Design review of the part built by this model. Coordinates are the model's own, in mm. Face numbers are marked on the shaded views. A direction names the side the tool comes from. Coordinates: 2 decimals unless noted, no trailing zeros. Write each loop counter-clockwise with the first axis right and the second up, starting at its lowest first coordinate (ties: lowest second). Pieces come first, ordered by that corner, then holes.
Q1. Take a section at A-A, the plane z = 7.75. Write out the cut boundary in (x, y).
Q2. For L1, parallel to Y at x = -13, z = 0.7; L2, parallel to X at y = -31, z = 13; L3, parallel to Y at x = 19.5, z = 3.75, list the stretches that pass through material, from the lowest coordinate up.
Q3. The part is to be moulded in two halves that separate along Y. For the marked faces 3, 4 and 5, say which applies: released by +Y, released by -Y, zero draft, split by the parting line, or undercut.
Q4. Take a section at B-B, the plane y = 16.5. Write out the cut boundary in (x, z), plus the area to 3 significant figures.
Q5. For the marked faces 1 and 2, list the 3-axis set-ups (+Z, -Z, +X, -X, +Y, -Y) from which the entire face can be reached by the end or side of a thin tool; tool diameter is ignored.
Q6. For pin 1 Ø3.5 at (x, z) = (-6, 7) entering from +Y; pin 2 Ø2 at (x, z) = (14.5, 9.5) entering from -Y; pin 3 Ø3 at (x, y) = (-12, 26.5) entering from +Z, all flat-tipped, find the tip position at first contact; note any pin that passes through.
Q7. Take a section at C-C, the plane x = -12.5. State how many separate pieces and enclosed holes the cut face has, plus the area to 3 significant figures.
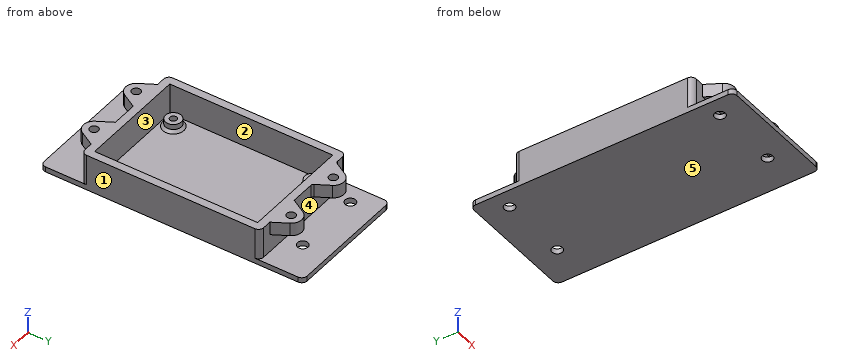
from build123d import *

# Parameters (mm, degrees)
SKETCH_1_W               = 40
SKETCH_1_H               = 100
SKETCH_1_R               = 2
EXTRUDE_1_DEPTH          = 2
SKETCH_2_W               = 47
SKETCH_2_H               = 68
SKETCH_2_W_2             = 41
SKETCH_2_H_2             = 62
EXTRUDE_2_DEPTH          = 11.8
SKETCH_3_W               = 7
SKETCH_3_H               = 100
EXTRUDE_3_DEPTH          = 2
SKETCH_4_R               = 3
SKETCH_4_R_2             = 1.3
EXTRUDE_4_DEPTH          = 3
SKETCH_5_R               = 1.3
CUT_EXTRUDE_1_DEPTH      = 3.5
SKETCH_6_R               = 1.65
EXTRUDE_5_DEPTH          = 5
CUT_EXTRUDE_2_DEPTH      = 2
FILLET_1_R               = 1
MIRROR_5_COPY_1_SKETCH_R = 1.65
MIRROR_5_COPY_1_DEPTH    = 5
MIRROR_5_COPY_2_DEPTH    = 2
FILLET_2_R               = 2
CHAMFER_1_SIZE           = 1


with BuildPart() as part:
    # 草图1 → 凸台-拉伸1 (new body)
    with BuildSketch(Plane.XY):
        Rectangle(SKETCH_1_W, SKETCH_1_H)
        with Locations((-13, 40)):
            Circle(SKETCH_1_R, mode=Mode.SUBTRACT)
        with Locations((13, 40)):
            Circle(SKETCH_1_R, mode=Mode.SUBTRACT)
        with Locations((-13, -40)):
            Circle(SKETCH_1_R, mode=Mode.SUBTRACT)
        with Locations((13, -40)):
            Circle(SKETCH_1_R, mode=Mode.SUBTRACT)
    extrude(amount=EXTRUDE_1_DEPTH)

    # 草图2 → 凸台-拉伸2 (add)
    with BuildSketch(Plane.XY.offset(2)):
        with Locations((3.5, -0.496887342)):
            Rectangle(SKETCH_2_W, SKETCH_2_H)
        with Locations((3.5, -0.496887342)):
            Rectangle(SKETCH_2_W_2, SKETCH_2_H_2, mode=Mode.SUBTRACT)
    extrude(amount=EXTRUDE_2_DEPTH)

    # 草图3 → 凸台-拉伸3 (add)
    with BuildSketch(Plane(origin=(0, 0, 0), x_dir=(-1, 0, 0), z_dir=(0, 0, -1))):
        with Locations((-23.5, 0)):
            Rectangle(SKETCH_3_W, SKETCH_3_H)
    extrude(amount=-EXTRUDE_3_DEPTH)

    # 草图4 → 凸台-拉伸4 (add)
    with BuildSketch(Plane.XY.offset(2)):
        with Locations(Location((-12.5, 26.003112658, 0), (0, 0, 180))):
            Circle(SKETCH_4_R)
        with Locations((-12.5, 26.003112658)):
            Circle(SKETCH_4_R_2, mode=Mode.SUBTRACT)
        with Locations(Location((19.5, 26.003112658, 0), (0, 0, 180))):
            Circle(SKETCH_4_R)
        with Locations((19.5, 26.003112658)):
            Circle(SKETCH_4_R_2, mode=Mode.SUBTRACT)
        with Locations(Location((19.5, -26.996887342, 0), (0, 0, 180))):
            Circle(SKETCH_4_R)
        with Locations((19.5, -26.996887342)):
            Circle(SKETCH_4_R_2, mode=Mode.SUBTRACT)
        with Locations(Location((-12.5, -26.996887342, 0), (0, 0, 180))):
            Circle(SKETCH_4_R)
        with Locations((-12.5, -26.996887342)):
            Circle(SKETCH_4_R_2, mode=Mode.SUBTRACT)
    extrude(amount=EXTRUDE_4_DEPTH)

    # 草图5 → 切除-拉伸1 (cut)
    with BuildSketch(Plane.XY.offset(5)):
        with Locations((-12.5, -26.996887342)):
            Circle(SKETCH_5_R)
        with Locations((19.5, -26.996887342)):
            Circle(SKETCH_5_R)
        with Locations((19.5, 26.003112658)):
            Circle(SKETCH_5_R)
        with Locations((-12.5, 26.003112658)):
            Circle(SKETCH_5_R)
    extrude(amount=-CUT_EXTRUDE_1_DEPTH, mode=Mode.SUBTRACT)

    # 草图6 → 凸台-拉伸5 (add)
    with BuildSketch(Plane.XY.offset(13.8)):
        with BuildLine():
            Line((-14.639528096, 33.503112658), (-1.360471904, 33.503112658))
            Line((-1.360471904, 33.503112658), (-4.535898385, 39.003112658))
            ThreePointArc((-4.535898385, 39.003112658), (-8, 41.003112658), (-11.464101615, 39.003112658))
            Line((-11.464101615, 39.003112658), (-14.639528096, 33.503112658))
        make_face()
        with Locations((-8, 37.003112658)):
            Circle(SKETCH_6_R, mode=Mode.SUBTRACT)
    extrude_5 = extrude(amount=-EXTRUDE_5_DEPTH)

    # 草图7 → 切除-拉伸2 (cut)
    with BuildSketch(Plane(origin=(0, 0, 8.8), x_dir=(-1, 0, 0), z_dir=(0, 0, -1))):
        Polygon((6.325684219, 39.903112658), (4.651368439, 37.003112658), (6.325684219, 34.103112658), (9.674315781, 34.103112658), (11.348631561, 37.003112658), (9.674315781, 39.903112658), align=None)
    cut_extrude_2 = extrude(amount=-CUT_EXTRUDE_2_DEPTH, mode=Mode.SUBTRACT)

    # 圆角1
    fillet_1_edges = [part.edges().sort_by_distance(p)[0] for p in [
        (-14.639528096, 33.503112658, 11.3),
        (-1.360471904, 33.503112658, 11.3),
    ]]
    fillet(fillet_1_edges, radius=FILLET_1_R)

    # 镜向1: 凸台-拉伸5, 切除-拉伸2 across plane
    add(extrude_5.mirror(Plane(origin=(3.5, 0, 0), x_dir=(0, 0, 1), z_dir=(1, 0, 0))))
    add(cut_extrude_2.mirror(Plane(origin=(3.5, 0, 0), x_dir=(0, 0, 1), z_dir=(1, 0, 0))), mode=Mode.SUBTRACT)

    # 镜向5: 凸台-拉伸5, 切除-拉伸2 across plane
    add(extrude_5.mirror(Plane(origin=(0, -0.496887342, 0), x_dir=(0, 0, 1), z_dir=(0, -1, 0))))
    add(cut_extrude_2.mirror(Plane(origin=(0, -0.496887342, 0), x_dir=(0, 0, 1), z_dir=(0, -1, 0))), mode=Mode.SUBTRACT)

    # 镜向5 copy 1 sketch → 镜向5 copy 1 (add)
    with BuildSketch(Plane(origin=(7, -0.993774684, 13.8), x_dir=(-1, 0, 0), z_dir=(0, 0, 1))):
        with BuildLine():
            Line((-14.639528096, 33.503112658), (-1.360471904, 33.503112658))
            Line((-1.360471904, 33.503112658), (-4.535898385, 39.003112658))
            ThreePointArc((-4.535898385, 39.003112658), (-8, 41.003112658), (-11.464101615, 39.003112658))
            Line((-11.464101615, 39.003112658), (-14.639528096, 33.503112658))
        make_face()
        with Locations((-8, 37.003112658)):
            Circle(MIRROR_5_COPY_1_SKETCH_R, mode=Mode.SUBTRACT)
    extrude(amount=-MIRROR_5_COPY_1_DEPTH)

    # 镜向5 copy 2 sketch → 镜向5 copy 2 (cut)
    with BuildSketch(Plane(origin=(7, -0.993774684, 8.8), x_dir=(1, 0, 0), z_dir=(0, 0, -1))):
        Polygon((6.325684219, 39.903112658), (4.651368439, 37.003112658), (6.325684219, 34.103112658), (9.674315781, 34.103112658), (11.348631561, 37.003112658), (9.674315781, 39.903112658), align=None)
    extrude(amount=-MIRROR_5_COPY_2_DEPTH, mode=Mode.SUBTRACT)

    # 圆角2
    fillet_2_edges = [part.edges().sort_by_distance(p)[0] for p in [
        (27, 33.503112658, 7.9),
        (-20, 33.503112658, 7.9),
        (-20, -34.496887342, 7.9),
        (27, -34.496887342, 7.9),
        (27, -50, 1),
        (27, 50, 1),
        (-20, -50, 1),
        (-20, 50, 1),
    ]]
    fillet(fillet_2_edges, radius=FILLET_2_R)

    # 倒角1
    chamfer_1_edges = [part.edges().sort_by_distance(p)[0] for p in [
        (-9.5, 26.003112658, 2),
        (22.5, 26.003112658, 2),
        (22.5, -26.996887342, 2),
        (-9.5, -26.996887342, 2),
    ]]
    chamfer(chamfer_1_edges, length=CHAMFER_1_SIZE)


solid = part.part
Responses:
1. outline: (-20, -32.5) arc R2 ccw to (-18, -34.5) - (25, -34.5) arc R2 ccw to (27, -32.5) - (27, 31.5) arc R2 ccw to (25, 33.5) - (-18, 33.5) arc R2 ccw to (-20, 31.5) - close; hole (-17, -31.5) - (24, -31.5) - (24, 30.5) - (-17, 30.5) - close
2. L1: y = -50 to -42, -38 to 38, 42 to 50
2. L2: x = -20 to -17, 24 to 27
2. L3: y = -34.5 to -31.5, -30 to -28.3, -25.7 to -24, 23 to 24.7, 27.3 to 29, 30.5 to 33.5
3. face 3: undercut
3. face 4: released by +Y
3. face 5: zero draft
4. outline: (-20, 0) - (27, 0) - (27, 13.8) - (24, 13.8) - (24, 2) - (-17, 2) - (-17, 13.8) - (-20, 13.8) - close
4. area: 165 mm2
5. face 1: +Z, -Z, +X, +Y, -Y
5. face 2: +Z
6. pin 1: stops at y = 33.5
6. pin 2: stops at y = -42
6. pin 3: stops at z = 5
7. separate pieces: 3
7. enclosed holes: 0
7. area: 312 mm2
